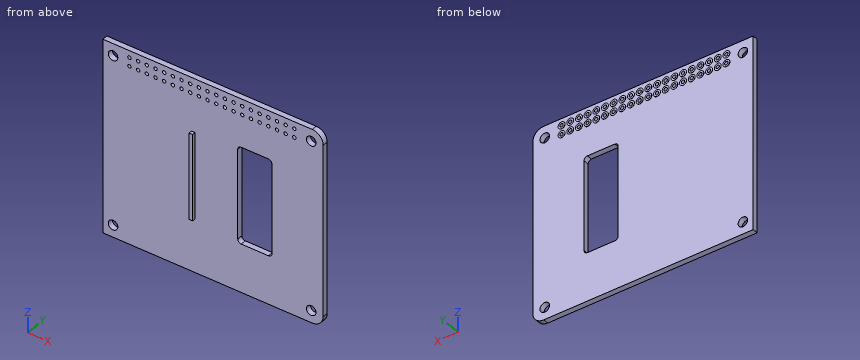
from build123d import *

# Parameters (mm, degrees)
SKETCH1_R            = 1.4
BOSS_EXTRUDE1_DEPTH  = 1.6
SKETCH2_R            = 0.5
CUT_EXTRUDE1_DEPTH   = 43.739004434
BOSS_EXTRUDE2_START  = 0.05
SKETCH3_R            = 1
SKETCH3_R_2          = 0.5
BOSS_EXTRUDE2_DEPTH  = 0.05
LPATTERN1_COUNT      = 20
LPATTERN1_PITCH      = 2.54
LPATTERN1_COUNT_DIR2 = 2
LPATTERN1_PITCH_DIR2 = 2.54
SKETCH4_W            = 1
SKETCH4_H            = 25
BOSS_EXTRUDE3_DEPTH  = 1


with BuildPart() as part:
    # Sketch1 → Boss-Extrude1 (new body)
    with BuildSketch(Plane(origin=(0, 0, 0), x_dir=(1, 0, 0), z_dir=(0, 1, 0))):
        with BuildLine():
            Line((-32.25, -28), (29.05, -28))
            ThreePointArc((29.05, -28), (31.3127417, -27.0627417), (32.25, -24.8))
            Line((32.25, -24.8), (32.25, 24.8))
            ThreePointArc((32.25, 24.8), (31.3127417, 27.0627417), (29.05, 28))
            Line((29.05, 28), (-32.25, 28))
            Line((-32.25, 28), (-32.25, -28))
        make_face()
        with Locations(Location((-29.25, -24.5, 0), (0, 0, 270))):
            Circle(SKETCH1_R, mode=Mode.SUBTRACT)
        with Locations(Location((-29.25, 24.5, 0), (0, 0, 270))):
            Circle(SKETCH1_R, mode=Mode.SUBTRACT)
        with Locations(Location((28.75, 24.5, 0), (0, 0, 270))):
            Circle(SKETCH1_R, mode=Mode.SUBTRACT)
        with Locations(Location((28.75, -24.5, 0), (0, 0, 270))):
            Circle(SKETCH1_R, mode=Mode.SUBTRACT)
        with BuildLine():
            Line((16.25, -14), (8.25, -14))
            ThreePointArc((8.25, -14), (7.542893219, -13.707106781), (7.25, -13))
            Line((7.25, -13), (7.25, 13))
            ThreePointArc((7.25, 13), (7.542893219, 13.707106781), (8.25, 14))
            Line((8.25, 14), (16.25, 14))
            ThreePointArc((16.25, 14), (16.957106781, 13.707106781), (17.25, 13))
            Line((17.25, 13), (17.25, -13))
            ThreePointArc((17.25, -13), (16.957106781, -13.707106781), (16.25, -14))
        make_face(mode=Mode.SUBTRACT)
    extrude(amount=BOSS_EXTRUDE1_DEPTH)

    # Sketch2 → Cut-Extrude1 (cut, through all)
    with BuildSketch(Plane(origin=(0, 1.6, 0), x_dir=(1, 0, 0), z_dir=(0, 1, 0))):
        with Locations(Location((-24.45, -26, 0), (0, 0, 270))):
            Circle(SKETCH2_R)
    cut_extrude1 = extrude(amount=-CUT_EXTRUDE1_DEPTH, mode=Mode.SUBTRACT)

    # Sketch3 → Boss-Extrude2 (add)
    with BuildSketch(Plane(origin=(0, 1.6, 0), x_dir=(1, 0, 0), z_dir=(0, 1, 0)).offset(BOSS_EXTRUDE2_START)):
        with Locations(Location((-24.45, -26, 0), (0, 0, 90))):
            Circle(SKETCH3_R)
        with Locations(Location((-24.45, -26, 0), (0, 0, 270))):
            Circle(SKETCH3_R_2, mode=Mode.SUBTRACT)
    boss_extrude2 = extrude(amount=-BOSS_EXTRUDE2_DEPTH)

    # LPattern1: Cut-Extrude1, Boss-Extrude2 20 × 2
    with Locations(*[(i * LPATTERN1_PITCH, 0, -j * LPATTERN1_PITCH_DIR2) for i in range(LPATTERN1_COUNT) for j in range(LPATTERN1_COUNT_DIR2) if (i, j) != (0, 0)]):
        add(cut_extrude1, mode=Mode.SUBTRACT)
        add(boss_extrude2)

    # Sketch4 → Boss-Extrude3 (add)
    with BuildSketch(Plane.XZ):
        with Locations((-5.75, 0)):
            Rectangle(SKETCH4_W, SKETCH4_H)
    extrude(amount=BOSS_EXTRUDE3_DEPTH)


solid = part.part
For this review, take the finished solid that the model builds, in its own axes (mm). Coordinates: 2 decimals unless noted, no trailing zeros. Loops run counter-clockwise (first coordinate to the right, second up) from the corner with the lowest first, then second, coordinate; pieces in that order, holes last. Notation, with made-up numbers: (66, 3) -> (119, 3) arc R33 ccw to (119, 39) -> close; hole circle Ø3 at (-36, 73.5). An arc over 180 degrees is marked (long way). Write each question's results on one line, items separated by ' | '.
Q1. For pin 1 Ø1.7 at (x, z) = (-29.25, -24.5) entering from +Y; pin 2 Ø0.5 at (y, z) = (-0.5, 2.5) entering from +X; pin 3 Ø0.8 at (x, y) = (-5.5, -0.5) entering from -Z; pin 4 Ø4 at (x, z) = (25, -18.5) entering from +Y, all flat-tipped, find the tip position at first contact; note any pin that passes through.
Taken from the geometry:
pin 1: through | pin 2: x = -5.25 | pin 3: z = -12.5 | pin 4: y = 1.6
Q2. Add section A-A, the plane z = -6. State the section outline as (x, y) points, then the cut area to 3 significant figures.
Taken from the geometry:
outline: (-32.25, 0) -> (-6.25, 0) -> (-6.25, -1) -> (-5.25, -1) -> (-5.25, 0) -> (7.25, 0) -> (7.25, 1.6) -> (-32.25, 1.6) -> close; (17.25, 0) -> (32.25, 0) -> (32.25, 1.6) -> (17.25, 1.6) -> close | area: 88.2 mm²
Q3. To check wall thickness, follow line 1 along X through (y, z) = (0.7, -3); line 2 along Z through (x, y) = (14.5, 0.2); line 3 along Z through (x, y) = (-28, 0.45). State the ranges of each line that lie inside material, in increasing order. Write a range as [from, to].
Taken from the geometry:
line 1: [-32.25, 7.25], [17.25, 32.25] | line 2: [-28, -14], [14, 28] | line 3: [-28, -25.13], [-23.87, 23.87], [25.13, 28]
Q4. Add section B-B, the plane z = -15. State the section outline as (x, y) points, then the cut area to 3 significant figures.
Taken from the geometry:
outline: (-32.25, 0) -> (32.25, 0) -> (32.25, 1.6) -> (-32.25, 1.6) -> close | area: 103 mm²
